Autodesk Inventor part; units mm, degrees
ref_plane "YZ Plane" through (0, 0, 0) normal (1, 0, 0) x (0, 1, 0)
ref_plane "XZ Plane" through (0, 0, 0) normal (0, 1, 0) x (-1, 0, 0)
ref_plane "XY Plane" through (0, 0, 0) normal (0, 0, 1) x (1, 0, 0)
sketch "Sketch1" plane through (0, 0, 0) normal (0, 0, 1) x (1, 0, 0)
  line L0 (0, 0) -> (17, 0)
  line L1 (17, 0.8671) -> (17, 6)
  line L2 (15, 8) -> (2, 8)
  line L3 (0, 6) -> (0, 0)
  line L4 (17, -0.8671) -> (2, -4.8546)
  line L5 (2, -4.8546) -> (1.9259, -4.5758)
  line L6 (1.9259, -4.5758) -> (16.4929, -0.7033)
  arc A0 (17, -0.8671) -> (17, 0.8671) centre (17, 0) ccw
  arc A1 (16.1329, 0) -> (16.4929, -0.7033) centre (17, 0) ccw
  arc A2 (2, 8) -> (0, 6) centre (2, 6) ccw
  arc A3 (17, 6) -> (15, 8) centre (15, 6) ccw
  point P0 (17, 8)
  point P1 (0, 8)
  dimension "d0" = 17
  dimension "d1" = 8
  dimension "d9" = 2
extrude "Extrusion1" add sketch "Sketch1" along normal blind 5
sketch "Sketch2" plane through (0, 0, 5) normal (0, 0, 1) x (1, 0, 0)
  circle A0 centre (3.5, 3.5) radius 1.75
  circle A1 centre (13.3, 3.5) radius 1.75
  line L0 (0, 0) -> (16.1329, 0)
  line L1 (0, 6) -> (0, 0)
  dimension "d4" = 3.5
  dimension "d5" = 3.5
  dimension "d6" = 9.8
  dimension "d10" = 3.5
  dimension "d11" = 3.5
  dimension "d12" = 3.5
extrude "Extrusion2" cut sketch "Sketch2" against normal blind 5
equation "\"BendRadius\" = Thickness"
equation "\"BendReliefWidth\" = Thickness"
equation "\"BendReliefDepth\" = 0.5 * Thickness"
equation "\"CornerReliefSize\" = 4 * Thickness"
equation "\"MinimumRemnant\" = 2 * Thickness"
equation "\"TransitionRadius\" = BendRadius"
equation "\"JacobiRadiusSize\" = BendRadius"
equation "\"GapSize\" = Thickness"
properties part number "công tắc hành trình"
Part model, mm, in its own coordinate system. A direction names the side the tool comes from. Give positions to 0.01 mm unless a question says otherwise; leave off trailing zeros. Write each loop counter-clockwise with the first axis right and the second up, starting at its lowest first coordinate (ties: lowest second). Pieces come first, ordered by that corner, then holes.
1) Pin check, flat tip, straight feed: pin 1 (1 mm diameter, centred on y = 2.5, z = 1, fed in from +X). Stop position of the tip, or through.
Resolved:
pin 1: stops at x = 17
2) Cut at C-C on x = 13.75. Write the cut outline in (y, z), then the cut area to 3 significant figures.
Resolved:
outline: (-1.73, 0) - (-1.43, 0) - (-1.43, 5) - (-1.73, 5) - close; (0, 0) - (1.81, 0) - (1.81, 5) - (0, 5) - close; (5.19, 0) - (8, 0) - (8, 5) - (5.19, 5) - close
area: 24.6 mm2
3) Which spindle directions (+Z, -Z, +X, -X, +Y, -Y) get a long thin tool onto all of the face, cutting with end or side? Do faces 1 (the face through (8, 0, 2)), 2 (the face through (14.11, 1.95, 2.54)). Say none if no direction does.
Resolved:
face 1: +Z, -Z, -X
face 2: +Z, -Z
4) Cut at B-B on z = 1.85. Write the cut outline in (x, y), then the cut area to 3 significant figures.
Resolved:
outline: (0, 0) - (16.13, 0) arc R0.87 ccw to (16.49, -0.7) - (1.93, -4.58) - (2, -4.85) - (17, -0.87) arc R0.87 ccw to (17, 0.87) - (17, 6) arc R2 ccw to (15, 8) - (2, 8) arc R2 ccw to (0, 6) - close; hole circle Ø3.5 at (3.5, 3.5); hole circle Ø3.5 at (13.3, 3.5)
area: 121 mm2
5) Probe L1, parallel to X at y = 2.75, z = 3.4; L2, parallel to X at y = 3, z = 1.05; L3, parallel to Y at x = 3.5, z = 2.95. List the from-to ranges inside material, lowest first.
Resolved:
L1: x = 0 to 1.92, 5.08 to 11.72, 14.88 to 17
L2: x = 0 to 1.82, 5.18 to 11.62, 14.98 to 17
L3: y = -4.46 to -4.16, 0 to 1.75, 5.25 to 8
6) Cut at A-A on y = 3.5. Write the cut outline in (x, z), then the cut area to 3 significant figures.
Resolved:
outline: (0, 0) - (1.75, 0) - (1.75, 5) - (0, 5) - close; (5.25, 0) - (11.55, 0) - (11.55, 5) - (5.25, 5) - close; (15.05, 0) - (17, 0) - (17, 5) - (15.05, 5) - close
area: 50.0 mm2
7) Two-plate mould, pull along X, no slides. Class faces 3 (the face through (17, 3, 2)), 4 (the face through (2.11, 2.44, 2.54)), 5 (the face through (9, 8, 2)): released by +X, released by -X, zero draft, split by the parting line, or undercut.
Resolved:
face 3: released by +X
face 4: undercut
face 5: zero draft
